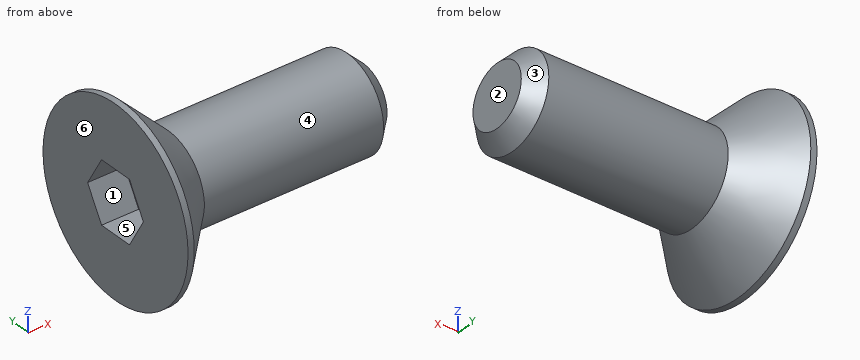
```python
from build123d import *

# Parameters (mm, degrees)
CHANFREIN1_SIZE         = 0.5
ENL_V_MAT_EXTRU_1_DEPTH = 1.2


with BuildPart() as part:
    # Esquisse1 → Révolution1 (revolve)
    with BuildSketch(Plane.XY):
        Polygon((0, 0), (0, 3), (0.2, 3), (1.7, 1.5), (8, 1.5), (8, 0), align=None)
    revolve(axis=Axis((8, 0, 0), (-1, 0, 0)))

    # Chanfrein1
    chanfrein1_edges = [part.edges().sort_by_distance(p)[0] for p in [
        (8, -1.5, 0),
    ]]
    chamfer(chanfrein1_edges, length=CHANFREIN1_SIZE)

    # Esquisse2 → Enlèv. mat.-Extru.1 (cut)
    with BuildSketch(Plane.ZY):
        Polygon((0, 1.154700538), (-1, 0.577350269), (-1, -0.577350269), (0, -1.154700538), (1, -0.577350269), (1, 0.577350269), align=None)
    extrude(amount=-ENL_V_MAT_EXTRU_1_DEPTH, mode=Mode.SUBTRACT)


solid = part.part
```
Input: part model. Units: mm. Frame: model coordinates. Face numbers are marked on the shaded views. A direction names the side the tool comes from. Coordinates: 2 decimals unless noted, no trailing zeros. Loops run counter-clockwise (first coordinate to the right, second up) from the corner with the lowest first, then second, coordinate; pieces in that order, holes last. Notation, with made-up numbers: (3, 31.25) - (56, 31.25) arc R17 ccw to (56, 52.25) - close; hole circle Ø11 at (31, 72.25). An arc over 180 degrees is marked (long way). Answer in a Markdown table with one row per item.
(1) Cut plane C-C on x = 3. Output: boundary loops of the cut face in (y, z).
Model answer:
| item | result |
|---|---|
| outline | circle Ø3 at (0, 0) |
(2) Mould query, pull axis Y, two halves, no side actions, for the marked faces 1, 2 and 3. Classes: pulls with the +Y half, pulls with the -Y half, needs draft (parallel to the pull), parting line crosses it, or undercut.
Model answer:
| item | result |
|---|---|
| face 1 | undercut |
| face 2 | needs draft |
| face 3 | parting line crosses it |
(3) Pin query (flat end, axial travel): P1, Ø2, axis at x = 1.5, z = 0.5, coming from the -Y side; P2, Ø2, axis at x = 2, y = 0, coming from the +Z side; P3, Ø2, axis at x = 3.5, y = 0.5, coming from the +Z side. Return the tip coordinate at first contact, or that it passes through.
Model answer:
| item | result |
|---|---|
| P1 | stops at y = -2.67 |
| P2 | stops at z = 2.2 |
| P3 | stops at z = 1.5 |
(4) Cut plane A-A on y = 0. Output: boundary loops of the cut face in (x, z), plus the area to 3 significant figures.
Model answer:
| item | result |
|---|---|
| outline | (0, -3) - (0.2, -3) - (1.7, -1.5) - (7.5, -1.5) - (8, -1) - (8, 1) - (7.5, 1.5) - (1.7, 1.5) - (0.2, 3) - (0, 3) - (0, 1) - (1.2, 1) - (1.2, -1) - (0, -1) - close |
| area | 24.2 mm² |
(5) Material intervals for L1, parallel to X at y = -0.85, z = -0.3; L2, parallel to Z at x = 1, y = -1.05; L3, parallel to Z at x = 0.75, y = 0.2, sorted ascending. Write a range as from..to.
Model answer:
| item | result |
|---|---|
| L1 | x = 1.2..8 |
| L2 | z = -1.93..-0.18, 0.18..1.93 |
| L3 | z = -2.44..-1, 1..2.44 |
(6) Cut plane B-B on x = 1. Output: boundary loops of the cut face in (y, z).
Model answer:
| item | result |
|---|---|
| outline | circle Ø4.4 at (0, 0); hole (-1.15, 0) - (-0.58, -1) - (0.58, -1) - (1.15, 0) - (0.58, 1) - (-0.58, 1) - close |
(7) Set-up query: the marked faces 4, 5 and 6. Return all of +Z, -Z, +X, -X, +Y, -Y with unobstructed straight access to the full face (end or side cutting, diameter ignored); none if empty.
Model answer:
| item | result |
|---|---|
| face 4 | +X |
| face 5 | -X |
| face 6 | +Z, -Z, -X, +Y, -Y |
